Autodesk Inventor part; units mm, degrees
ref_plane "YZ Plane" through (0, 0, 0) normal (1, 0, 0) x (0, 1, 0)
ref_plane "XZ Plane" through (0, 0, 0) normal (0, 1, 0) x (-1, 0, 0)
ref_plane "XY Plane" through (0, 0, 0) normal (0, 0, 1) x (1, 0, 0)
sketch "Sketch1" plane through (0, 0, 0) normal (0, 1, 0) x (-1, 0, 0)
  line L0 (18.5, 43) -> (-18.5, 43)
  line L1 (-18.5, 43) -> (-18.5, -43)
  line L2 (-18.5, -43) -> (18.5, -43)
  line L3 (18.5, -43) -> (18.5, 43)
  line L4 (18.5, 43) -> (-18.5, -43) construction
  line L5 (-18.5, 43) -> (18.5, -43) construction
  point P0 (0, 0)
  dimension "d0" = 37
  dimension "d1" = 86
extrude "Body" add sketch "Sketch1" along normal blind 11.2
sketch "Sketch2" plane through (18.5, 0, -43) normal (0, 0, -1) x (-1, 0, 0)
  circle A0 centre (32, 5) radius 1.85
  line L0 (37, 0) -> (37, 11.2)
  line L1 (0, 0) -> (37, 0)
  circle A1 centre (4.6, 5) radius 1.85
  line L2 (0, 0) -> (0, 11.2)
  point P0 (18.5, 0)
  dimension "d4" = 3.7
  dimension "d5" = 5
  dimension "d6" = 5
  dimension "d7" = 3.7
  dimension "d8" = 5
  dimension "d9" = 4.6
extrude "Side Mounts" cut sketch "Sketch2" against normal blind 11.2
sketch "Sketch3" plane through (0, 11.2, 0) normal (0, 1, 0) x (1, 0, 0)
  line L0 (-18.5, -43) -> (18.5, -43)
  line L1 (18.5, 43) -> (16, 43)
  line L2 (16, 43) -> (16, -43)
  line L3 (16, -43) -> (18.5, -43)
  line L4 (18.5, -43) -> (18.5, 43)
  line L5 (16, 40.5) -> (18.5, 40.5)
  point P0 (0, 0)
  point P1 (17.25, 43)
  point P2 (17.25, 40.5)
  dimension "d12" = 2.5
  dimension "d13" = 2.5
extrude "mains cutout" cut sketch "Sketch3" against normal up to surface (11.2 mm away) contours L2 L5 L4 L0
sketch "Sketch4" plane through (0, 11.2, 0) normal (0, 1, 0) x (1, 0, 0)
  line L0 (16, 40.5) -> (16, -43)
  line L1 (-18.5, -43) -> (-8.5, -43)
  line L2 (-8.5, -43) -> (-8.5, -18)
  line L3 (-8.5, -18) -> (16, -18)
  line L4 (16, -43) -> (-8.5, -43)
  point P0 (0, 0)
  dimension "d19" = 25
extrude "screen cut out" cut sketch "Sketch4" against normal up to surface (11.2 mm away)
sketch "Sketch5" plane through (0, 11.2, 0) normal (0, 1, 0) x (1, 0, 0)
  line L0 (-18.5524, -42.9481) -> (-17.2524, -42.9481)
  line L1 (-17.2524, -42.9481) -> (-17.2524, -32.9481)
  line L2 (-17.2524, -32.9481) -> (-18.5524, -32.9481)
  line L3 (-18.5524, -32.9481) -> (-18.5524, -42.9481)
  point P0 (0, 0)
  dimension "d22" = 1.3
  dimension "d23" = 10
extrude "top mount bracket" add sketch "Sketch5" along normal blind 9.5
sketch "Sketch6" plane through (-18.5524, 11.2, 32.9481) normal (-1, 0, 0) x (0, 0, 1)
  circle A0 centre (5, 5) radius 1.75
  line L0 (0, 9.5) -> (10, 9.5)
  line L1 (0, 0) -> (0, 9.5)
  line L2 (3.25, 5) -> (3.25, 9.5)
  line L3 (6.75, 9.5) -> (6.75, 5)
  point P0 (-32.9481, -11.2)
  dimension "d26" = 3.5
  dimension "d27" = 4.5
  dimension "d28" = 5
extrude "top mount hole" cut sketch "Sketch6" against normal up to surface (1.3 mm away)
sketch "Sketch7" plane through (0, 11.2, 0) normal (0, 1, 0) x (1, 0, 0)
  circle A0 centre (4.25, -4.5) radius 3.55
  line L0 (-18.5, 43) -> (-18.5, -32.9481)
  line L1 (-18.5, -43) -> (-8.5, -43)
  point P0 (0, 0)
  dimension "d32" = 7.1
  dimension "d33" = 22.75
  dimension "d34" = 38.5
extrude "Pot hole" cut sketch "Sketch7" against normal up to surface (11.2 mm away)
sketch "Sketch8" plane through (0, 11.2, 0) normal (0, 1, 0) x (1, 0, 0)
  circle A0 centre (4.25, -4.5) radius 9
  point P0 (0, 0)
  dimension "d37" = 18
extrude "Extrusion8" cut sketch "Sketch8" against normal blind 8
sketch "Sketch9" plane through (0, 11.2, 0) normal (0, 1, 0) x (1, 0, 0)
  line L0 (16, -18) -> (16, 40.5)
  line L1 (16, 40.5) -> (16, 28.5)
  line L2 (16, 40.5) -> (16, 36.5)
  line L3 (16, 36.5) -> (8, 36.5)
  line L4 (8, 36.5) -> (8, 24.5)
  line L5 (8, 24.5) -> (16, 24.5)
  line L6 (16, 24.5) -> (16, 36.5)
  point P0 (0, 0)
  dimension "d42" = 4
  dimension "d43" = 8
  dimension "d44" = 12
extrude "Extrusion9" cut sketch "Sketch9" against normal up to surface (11.2 mm away)
sketch "Sketch10" plane through (0, 11.2, 0) normal (0, 1, 0) x (1, 0, 0)
  line L0 (16, 36.5) -> (16, 40.5)
  line L1 (-17.2524, -32.9481) -> (-17.2524, -42.9481)
  line L2 (16, 36.5) -> (-17.2524, 36.5)
  line L3 (-17.2524, 36.5) -> (-17.2524, -42.9481)
  line L4 (-17.2524, -42.9481) -> (16, -42.9481)
  line L5 (16, -42.9481) -> (16, 36.5)
  point P0 (0, 0)
sketch "encoder locator" plane through (0, 0, 0) normal (0, -1, 0) x (1, 0, 0)
  line L0 (4.25, 4.5) -> (4.25, -1.5)
  circle A0 centre (4.25, -1.5) radius 1.75
  point P0 (0, 0)
  dimension "d49" = 6
  dimension "d50" = 3.5
extrude "Extrusion11" cut sketch "encoder locator" against normal up to surface (3.2 mm away)
equation "\"d8\" = d6"
properties part number "Knob Bracket v4_3DPrint"
The listing builds one solid part. Answer for the finished solid, in the listing's coordinates (mm). A direction names the side the tool comes from. Give positions to 0.01 mm unless a question says otherwise; leave off trailing zeros. Loops run counter-clockwise (first coordinate to the right, second up) from the corner with the lowest first, then second, coordinate; pieces in that order, holes last. Notation, with made-up numbers: M 43,66.25 L 88,66.25 A15 ccw 88,71.25 Z; hole C 5,7 d8. An arc over 180 degrees is marked long. Answer as CSV lines item,"result".
Item 1: The part is cut by section D-D (x = 4.25). Give the vertices of the cut face in (y, z), and give its area (3 significant figures).
Values follow:
outline,"M 0,-43 L 11.2,-43 L 11.2,-4.5 L 3.2,-4.5 L 3.2,-3.25 L 0,-3.25 Z; M 0,0.25 L 3.2,0.25 L 3.2,0.95 L 0,0.95 Z; M 0,8.05 L 3.2,8.05 L 3.2,13.5 L 11.2,13.5 L 11.2,18 L 0,18 Z"
area,"505 mm^2"
Item 2: Which of the six approach directions +Z, -Z, +X, -X, +Y, -Y give full straight-line access (tool end or side, diameter ignored) to faces 1 (the flat face through (16, 6, -4)), 2 (the flat face through (4.1, 3.2, 8.4)), 3 (the flat face through (8, 6, -31)), 4 (the cylindrical face through (-15.265, 5.556, -37.478))?
Values follow:
face 1,"+Z, +X, +Y, -Y"
face 2,"+Y"
face 3,"+X, +Y, -Y"
face 4,"-Z"
Item 3: The part is cut by section B-B (z = 4.5). Give the vertices of the cut face in (x, y).
Values follow:
outline,"M -18.5,0 L 0.7,0 L 0.7,3.2 L -4.75,3.2 L -4.75,11.2 L -18.5,11.2 Z; M 7.8,0 L 16,0 L 16,11.2 L 13.25,11.2 L 13.25,3.2 L 7.8,3.2 Z"
Item 4: The part is cut by section C-C (y = 19). Give the vertices of the cut face in (x, z).
Values follow:
outline,"M -18.55,32.95 L -17.25,32.95 L -17.25,36.2 L -18.55,36.2 Z; M -18.55,39.7 L -17.25,39.7 L -17.25,42.95 L -18.55,42.95 Z"
Item 5: The mould has two halves that part along Z. Classify faces 5 (the cylindrical face through (7.53, 1.62, 5.86)), 6 (the flat face through (0, 6, -43)), 7 (the flat face through (-14, 6, 43)), 8 (the flat face through (-4, 0, -9)): released by +Z, released by -Z, zero draft, split by the parting line, or undercut.
Values follow:
face 5,"undercut"
face 6,"released by -Z"
face 7,"released by +Z"
face 8,"zero draft"
Item 6: The part is cut by section A-A (y = 5). Give the vertices of the cut face in (x, z), and give its area (3 significant figures).
Values follow:
outline,"M -18.5,-43 L -15.35,-43 L -15.35,-31.8 L -11.65,-31.8 L -11.65,-43 L 12.05,-43 L 12.05,-36.5 L 8,-36.5 L 8,-24.5 L 16,-24.5 L 16,18 L -8.5,18 L -8.5,43 L -18.5,43 Z; M 15.75,-43 L 18.5,-43 L 18.5,-40.5 L 16,-40.5 L 16,-36.5 L 15.75,-36.5 Z; hole C 4.25,4.5 d18"
area,"1,940 mm^2"
Item 7: Given pin 1 Ø9 at (x, z) = (4.25, 4.5) entering from +Y; pin 2 Ø4 at (x, y) = (5, 9) entering from +Z; pin 3 Ø1.2 at (x, y) = (17, 7) entering from +Z, each flat-ended and moving along its own axis, determine where each tip first touches the part or whether it passes through.
Values follow:
pin 1,"stops at y = 3.2"
pin 2,"stops at z = 18"
pin 3,"stops at z = -40.5"
Item 8: Straight lines are drawn through the part: line 1 along Z through (x, y) = (4.25, 1.1); line 2 along Z through (x, y) = (4.25, 5); line 3 along Z through (x, y) = (11, 7.75). For each, find the intervals that lie inside material, in ascending order. Write a range as [from, to].
Values follow:
line 1,"z = [-43, -3.25], [0.25, 0.95], [8.05, 18]"
line 2,"z = [-43, -4.5], [13.5, 18]"
line 3,"z = [-43, -36.5], [-24.5, -1.45], [10.45, 18]"
